Input: part model. Units: mm. Frame: model coordinates. A direction names the side the tool comes from. Give positions to 0.01 mm unless a question says otherwise; leave off trailing zeros. Order: outer loops, then holes, each group sorted by start corner. A loop starts at its lowest first (then second) coordinate and runs counter-clockwise, first axis right, second up. Notation, with made-up numbers: (2.25, 63) -> (29.25, 63) arc R13 cw to (29.25, 71) -> close; hole circle Ø9 at (78.25, 42). An arc over 180 degrees is marked (long way). Use a Markdown table: item, result. Add a question column.
from build123d import *

# Parameters (mm, degrees)
SALIENTE_EXTRUIR1_DEPTH = 30
CORTAR_EXTRUIR1_DEPTH   = 10


with BuildPart() as part:
    # Croquis1 → Saliente-Extruir1 (new body, symmetric)
    with BuildSketch(Plane(origin=(0, 0, 0), x_dir=(0, 0, -1), z_dir=(1, 0, 0))):
        Polygon((0, 0), (-60, 0), (-60, 20), (-40, 20), (-40, 40), (-20, 40), (-20, 60), (0, 60), align=None)
    extrude(amount=SALIENTE_EXTRUIR1_DEPTH, both=True)

    # Croquis2 → Cortar-Extruir1 (cut, symmetric)
    with BuildSketch(Plane(origin=(0, 0, 0), x_dir=(0, 0, -1), z_dir=(1, 0, 0))):
        Polygon((-40, 20), (-20, 40), (-40, 40), align=None)
        Polygon((-60, 0), (-40, 20), (-60, 20), align=None)
        Polygon((-20, 40), (0, 60), (-20, 60), align=None)
    extrude(amount=CORTAR_EXTRUIR1_DEPTH, both=True, mode=Mode.SUBTRACT)


solid = part.part
Q1. Section query C-C (x = 3.5). Return loops of the section in (y, z), plus the area to 3 significant figures.
Q2. Ray query, line 1 (X direction, y = 49, z = 17); line 2 (Z direction, x = 14, y = 40.5). Return the intervals inside material, ascending.
Q3. Draft query along X for faces 1 (the flat face through (30, 24, 23)), 2 (the flat face through (-20, 10, 60)), 3 (the flat face through (10, 32, 32)). Return one class per face: +X half, -X half, draft (parallel to the pull), parting line (faces both ways), or undercut.
Q4. First-contact query: pin 1 (10 mm diameter, centred on x = 25, z = 48, fed in from +Y); pin 2 (22 mm diameter, centred on x = -21, y = 33, fed in from +Z); pin 3 (6 mm diameter, centred on x = 17, z = 34.5, fed in from +Y). Flat tips, straight axial feed; report the tip coordinate or a pass-through.
Q5. Section query B-B (y = 52). Return loops of the section in (x, z), plus the area to 3 significant figures.
Q6. Access query for faces 4 (the flat face through (10, 12, 52)), 5 (the flat face through (-20, 50, 20)), 6 (the flat face through (-30, 24, 23)). Directions: +Z, -Z, +X, -X, +Y, -Y. A direction counts if a zero-diameter tool reaches every point of the face in a straight line with its end or side. Return the directions, or none.
Q7. Section query A-A (z = 37). Return loops of the section in (x, y).
Solution:
| question | item | result |
|---|---|---|
| 1 | outline | (0, 0) -> (60, 0) -> (0, 60) -> close |
| 1 | area | 1,800 mm² |
| 2 | line 1 | x = -30 to -10, 10 to 30 |
| 2 | line 2 | z = 0 to 20 |
| 3 | face 1 | +X half |
| 3 | face 2 | draft |
| 3 | face 3 | undercut |
| 4 | pin 1 | stops at y = 20 |
| 4 | pin 2 | stops at z = 40 |
| 4 | pin 3 | stops at y = 40 |
| 5 | outline | (-30, 0) -> (30, 0) -> (30, 20) -> (10, 20) -> (10, 8) -> (-10, 8) -> (-10, 20) -> (-30, 20) -> close |
| 5 | area | 960 mm² |
| 6 | face 4 | +Z, +Y |
| 6 | face 5 | +Z, +X, -X, +Y |
| 6 | face 6 | +Z, -Z, -X, +Y, -Y |
| 7 | outline | (-30, 0) -> (30, 0) -> (30, 40) -> (10, 40) -> (10, 23) -> (-10, 23) -> (-10, 40) -> (-30, 40) -> close |
